```python
from build123d import *

# Parameters (mm, degrees)
F0_W      = 150
F0_H      = 150
F1_DEPTH  = 10
F2_R      = 45
F3_DEPTH  = 280
F4_R      = 35
F5_DEPTH  = 280
F6_W      = 150
F6_H      = 150
F7_DEPTH  = 10
F8_R      = 7
F9_DEPTH  = 300.001
F10_R     = 4
F11_DEPTH = 25
F12_R     = 4
F13_DEPTH = 300.001


with BuildPart() as f1:
    # F0 (on Top) → F1 (new body)
    with BuildSketch(Plane.XY):
        with Locations((-2.5494610891, -9.9877563774)):
            Rectangle(F0_W, F0_H)
    extrude(amount=F1_DEPTH)

    # F2 (on face) → F3 (join)
    with BuildSketch(Plane.XY.offset(10)):
        with Locations((-2.5494610891, -9.9877563774)):
            Circle(F2_R)
    extrude(amount=F3_DEPTH)

    # F4 (on face) → F5 (cut)
    with BuildSketch(Plane.XY.offset(290)):
        with Locations((-2.5494610891, -9.9877563774)):
            Circle(F4_R)
    extrude(amount=-F5_DEPTH, mode=Mode.SUBTRACT)

    # F6 (on face) → F7 (join)
    with BuildSketch(Plane.XY.offset(290)):
        with Locations((-2.4832710624, -9.8278763674)):
            Rectangle(F6_W, F6_H)
    extrude(amount=F7_DEPTH)

    # F8 (on face) → F9 (cut, through all)
    with BuildSketch(Plane.XY.offset(300)):
        with Locations((-2.4832710624, -9.8278763674)):
            Circle(F8_R)
    extrude(amount=-F9_DEPTH, mode=Mode.SUBTRACT)

    # F10 (on face) → F11 (cut)
    with BuildSketch(Plane.XY.offset(300)):
        with Locations((-22.4832710624, -29.8278763674)):
            Circle(F10_R)
        with Locations((17.5167289376, 10.1721236326)):
            Circle(F10_R)
    extrude(amount=-F11_DEPTH, mode=Mode.SUBTRACT)

    # F12 (on face) → F13 (cut, through all)
    with BuildSketch(Plane.XY.offset(300)):
        with Locations((-2.4832710624, 45.1721236326)):
            Circle(F12_R)
        with Locations((-41.4732710624, 29.1621236326)):
            Circle(F12_R)
        with Locations((-57.4832710624, -9.9877563774)):
            Circle(F12_R)
        with BuildLine():
            ThreePointArc((-44.3345995739, -51.6792048789), (-39.9871328279, -52.5043756512), (-37.5394610891, -48.8178763674))
            ThreePointArc((-37.5394610891, -48.8178763674), (-37.8350506066, -47.3087895651), (-38.6781325776, -46.0227378826))
            ThreePointArc((-38.6781325776, -46.0227378826), (-44.3016981871, -46.0556392694), (-44.3345995739, -51.6792048789))
        make_face()
        with BuildLine():
            ThreePointArc((-38.6781325776, -46.0227378826), (-37.8350506066, -47.3087895651), (-37.5394610891, -48.8178763674))
            ThreePointArc((-37.5394610891, -48.8178763674), (-39.9871328279, -52.5043756512), (-44.3345995739, -51.6792048789))
            ThreePointArc((-44.3345995739, -51.6792048789), (-39.96418426, -52.5884768766), (-37.4732710624, -48.8840663941))
            ThreePointArc((-37.4732710624, -48.8840663941), (-37.7867717786, -47.331738133), (-38.6781325776, -46.0227378826))
        make_face()
        with BuildLine():
            ThreePointArc((-44.3345995739, -51.6792048789), (-44.3016981871, -46.0556392694), (-38.6781325776, -46.0227378826))
            ThreePointArc((-38.6781325776, -46.0227378826), (-44.3678882138, -45.9894492427), (-44.3345995739, -51.6792048789))
        make_face()
        with Locations((52.5167289376, -9.8278763674)):
            Circle(F12_R)
        with Locations((36.5067289376, -48.8178763674)):
            Circle(F12_R)
        with Locations((-2.6431510724, -64.8278763674)):
            Circle(F12_R)
        with Locations((36.5067289376, 29.2283136593)):
            Circle(F12_R)
    extrude(amount=-F13_DEPTH, mode=Mode.SUBTRACT)


solid = f1.part
```
Geometry: final body of the model. Coordinates: model frame, mm. A direction names the side the tool comes from. Round coordinates to 2 decimals unless told otherwise and drop trailing zeros. Loops run counter-clockwise (first coordinate to the right, second up) from the corner with the lowest first, then second, coordinate; pieces in that order, holes last. Notation, with made-up numbers: (43.5, 84.25) -> (68.5, 84.25) arc R21 ccw to (68.5, 121.25) -> close; hole circle Ø10 at (43.5, -30.75). An arc over 180 degrees is marked (long way). Use one line per item in the form item = value. Start each with the question number.
1) Section A-A on x = -21.5. Output: boundary loops of the cut face in (y, z), then the cut area to 3 significant figures.
2) First-contact query: P1, Ø11, axis at x = -2.48, y = -9.83, coming from the -Z side (3 decimals); P2, Ø11, axis at y = -38.5, z = 297, coming from the -X side; P3, Ø4, axis at x = 26, z = 55, coming from the -Y side; P4, Ø3, axis at x = -23.5, z = 251, coming from the -Y side. Flat tips, straight axial feed; report the tip coordinate or a pass-through.
3) Access query for faces 4 (the flat face through (-3, -17, 290)), 5 (the cylindrical face through (13.52, 10.35, 295.07)), 6 (the flat face through (-4, -84.988, 5)). Directions: +Z, -Z, +X, -X, +Y, -Y. A direction counts if a zero-diameter tool reaches every point of the face in a straight line with its end or side. Return the directions, or none.
4) Section B-B on x = 24.5. Output: boundary loops of the cut face in (y, z).
5) Line query: L1, parallel to Z at x = 45, y = 26; L2, parallel to Y at x = -3.5, z = 215.5; L3, parallel to Y at x = -16, z = 176.5. Output: solid intervals per line, ascending.
6) Section C-C on z = 230.5. Output: boundary loops of the cut face in (x, y).
7) Draft query along X for faces 1 (the flat face through (-4, 65.172, 295)), 2 (the flat face through (-77.483, -11, 295)), 3 (the cylindrical face through (40.32, 30.43, 295.07)). Return one class per face: released by +X, released by -X, zero draft, split by the parting line, or undercut.
Response:
q1.outline = (-84.99, 0) -> (65.01, 0) -> (65.01, 10) -> (30.83, 10) -> (30.83, 290) -> (65.17, 290) -> (65.17, 300) -> (-25.95, 300) -> (-25.95, 290) -> (19.44, 290) -> (19.44, 10) -> (-39.41, 10) -> (-39.41, 290) -> (-33.71, 290) -> (-33.71, 300) -> (-84.83, 300) -> (-84.83, 290) -> (-50.8, 290) -> (-50.8, 10) -> (-84.99, 10) -> close
q1.area = 9,300 mm^2
q2.P1 = through
q2.P2 = -77.48
q2.P3 = -46.32
q2.P4 = -50.57
q3.face_4 = none
q3.face_5 = +Z
q3.face_6 = +Z, -Z, +X, -X, -Y
q4.outline = (-84.99, 0) -> (65.01, 0) -> (65.01, 10) -> (25.98, 10) -> (25.98, 290) -> (65.17, 290) -> (65.17, 300) -> (-84.83, 300) -> (-84.83, 290) -> (-45.95, 290) -> (-45.95, 10) -> (-84.99, 10) -> close; hole (-32.2, 10) -> (12.22, 10) -> (12.22, 290) -> (-32.2, 290) -> close
q5.L1 = 0 to 10, 290 to 300
q5.L2 = -54.98 to -44.97, 25 to 35
q5.L3 = -52.93 to -42.3, 22.32 to 32.96
q6.outline = circle Ø90 at (-2.55, -9.99); hole circle Ø70 at (-2.55, -9.99)
q7.face_1 = zero draft
q7.face_2 = released by -X
q7.face_3 = undercut
